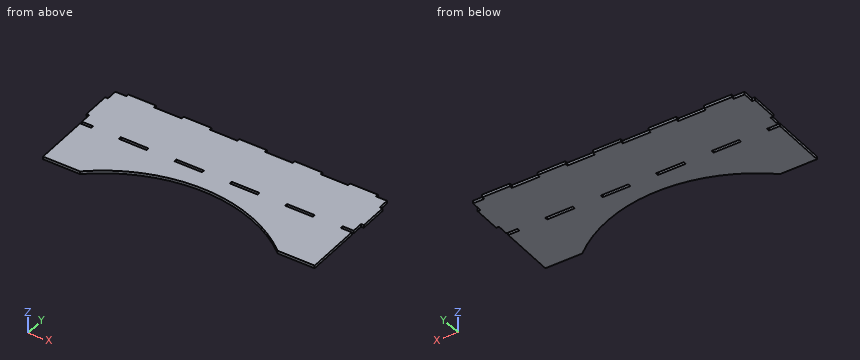
```python
from build123d import *

# Parameters (mm, degrees)
SKETCH1_W           = 300
SKETCH1_H           = 60
BOSS_EXTRUDE1_DEPTH = 3
SKETCH3_W           = 300
SKETCH3_H           = 60
BOSS_EXTRUDE2_DEPTH = 3
SKETCH2_W           = 30
SKETCH2_H           = 3
CUT_EXTRUDE6_DEPTH  = 5
SKETCH4_W           = 3
SKETCH4_H           = 60
CUT_EXTRUDE7_DEPTH  = 5


with BuildPart() as part:
    # Sketch1 → Boss-Extrude1 (new body)
    with BuildSketch(Plane.XY):
        with Locations((150, 30)):
            Rectangle(SKETCH1_W, SKETCH1_H)
    extrude(amount=BOSS_EXTRUDE1_DEPTH)

    # Sketch3 → Boss-Extrude2 (add)
    with BuildSketch(Plane.XY.offset(3)):
        with Locations((150, -30)):
            Rectangle(SKETCH3_W, SKETCH3_H)
    extrude(amount=-BOSS_EXTRUDE2_DEPTH)

    # Sketch2 → Cut-Extrude6 (cut)
    with BuildSketch(Plane.XY.offset(3)):
        Polygon((15, 0), (15, 3), (3, 3), (3, 15), (0, 15), (0, 0), align=None)
        with Locations((60, 1.5)):
            Rectangle(SKETCH2_W, SKETCH2_H)
        with Locations((120, 1.5)):
            Rectangle(SKETCH2_W, SKETCH2_H)
        with Locations((180, 1.5)):
            Rectangle(SKETCH2_W, SKETCH2_H)
        with Locations((240, 1.5)):
            Rectangle(SKETCH2_W, SKETCH2_H)
        Polygon((300, 0), (300, 15), (297, 15), (297, 3), (285, 3), (285, 0), align=None)
        Polygon((300, 45), (300, 60), (285, 60), (285, 57), (297, 57), (297, 45), align=None)
        with Locations((240, 58.5)):
            Rectangle(SKETCH2_W, SKETCH2_H)
        with Locations((180, 58.5)):
            Rectangle(SKETCH2_W, SKETCH2_H)
        with Locations((120, 58.5)):
            Rectangle(SKETCH2_W, SKETCH2_H)
        with Locations((60, 58.5)):
            Rectangle(SKETCH2_W, SKETCH2_H)
        Polygon((0, 60), (0, 45), (3, 45), (3, 57), (15, 57), (15, 60), align=None)
    extrude(amount=-CUT_EXTRUDE6_DEPTH, mode=Mode.SUBTRACT)

    # Sketch4 → Cut-Extrude7 (cut)
    with BuildSketch(Plane.XY.offset(3)):
        with Locations((1.5, -30)):
            Rectangle(SKETCH4_W, SKETCH4_H)
        with Locations((298.5, -30)):
            Rectangle(SKETCH4_W, SKETCH4_H)
        with BuildLine():
            Line((43, -60), (257, -60))
            ThreePointArc((257, -60), (150, -20), (43, -60))
        make_face()
    extrude(amount=-CUT_EXTRUDE7_DEPTH, mode=Mode.SUBTRACT)


solid = part.part
```
The model under review builds one solid part; all positions refer to its coordinate system, in mm. Round coordinates to 2 decimals unless told otherwise and drop trailing zeros. Write each loop counter-clockwise with the first axis right and the second up, starting at its lowest first coordinate (ties: lowest second). Pieces come first, ordered by that corner, then holes.
(1) We need section D-D on y = -5. Give the boundary of the cut face in (x, z), and give its area (3 significant figures).
(2) We need section B-B on y = -51. Give the boundary of the cut face in (x, z), and give its area (3 significant figures).
(3) Insertion check: pin 1 (1.5 mm diameter, centred on y = 58.5, z = 2, fed in from +X); pin 2 (1.5 mm diameter, centred on x = 1, z = 1.5, fed in from -Y); pin 3 (1.5 mm diameter, centred on x = 169.5, z = 2.5, fed in from -Y). Each pin has a flat end and moves straight along its axis. Give the tip position at first contact, or say it passes through.
(4) We need section C-C on z = 0.85. Give the number of separate pieces and of enclosed holes in the cut face, and give its area (3 significant figures).
(5) We need section A-A on x = 114.5. Give the boundary of the cut face in (y, z), and give its area (3 significant figures).
(6) Wall thickness on L1, parallel to X at y = 49.5, z = 2.35; L2, parallel to Y at x = 50.5, z = 2.35; L3, parallel to Y at x = 194, z = 1.6: over which ranges is each line inside the solid? List them lowest first.
Findings below:
1. outline: (3, 0) - (297, 0) - (297, 3) - (3, 3) - close
1. area: 882 mm2
2. outline: (3, 0) - (54.33, 0) - (54.33, 3) - (3, 3) - close; (245.67, 0) - (297, 0) - (297, 3) - (245.67, 3) - close
2. area: 308 mm2
3. pin 1: stops at x = 285
3. pin 2: stops at y = 15
3. pin 3: stops at y = -21.26
4. separate pieces: 1
4. enclosed holes: 4
4. area: 28,700 mm2
5. outline: (-23.91, 0) - (0, 0) - (0, 3) - (-23.91, 3) - close; (3, 0) - (57, 0) - (57, 3) - (3, 3) - close
5. area: 234 mm2
6. L1: x = 3 to 297
6. L2: y = -53.86 to 0, 3 to 57
6. L3: y = -26.05 to 0, 3 to 57
